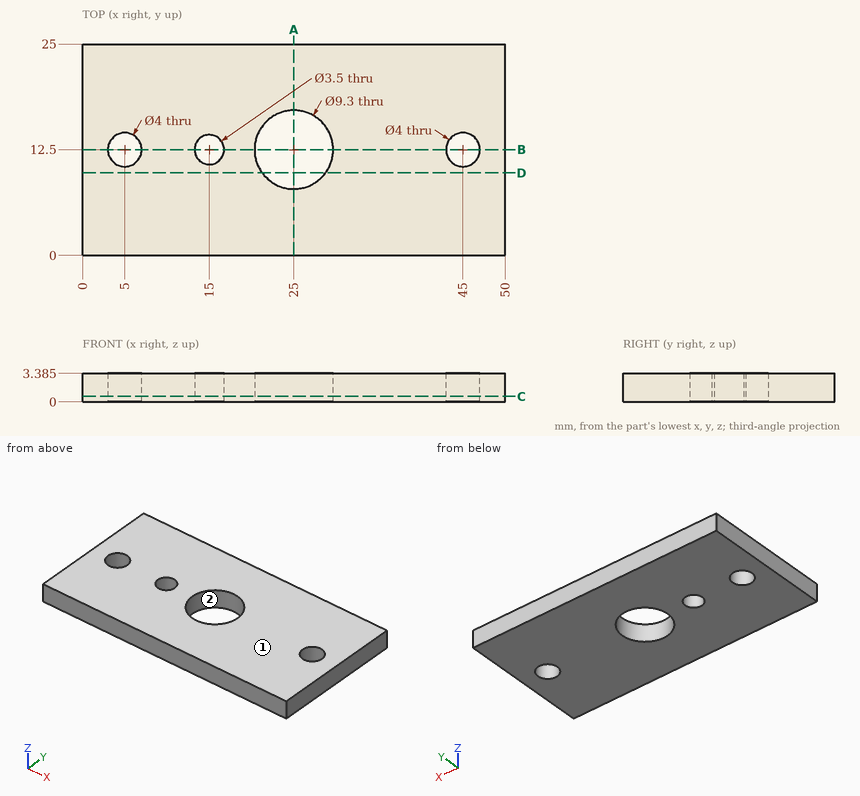
Check sheet for the drawn part. Datum: minimum x, y, z corner. Units: mm. Coordinates: 2 decimals unless noted, no trailing zeros. Order: outer loops, then holes, each group sorted by start corner. A loop starts at its lowest first (then second) coordinate and runs counter-clockwise, first axis right, second up. Notation, with made-up numbers: M 83.5,-7.75 L 132.5,-7.75 A13 cw 132.5,-3.75 Z; hole C -37,-40 d11. An arc over 180 degrees is marked long. One line per item, written item: value. Start each with the question number.
Item 1: Mould release check, pull along X, two halves, no side actions. Record for the marked faces 1 and 2: released by +X, released by -X, zero draft, split by the parting line, or undercut.
Item 2: Sectioned sample at C-C (z = 0.65). Enter the section's corners in (x, y), then the cut area to 3 significant figures.
Item 3: Gauge pin test, flat end, axial feed: pin 1 (5.5 mm diameter, centred on x = 15, y = 12.5, fed in from -Z). Record the tip position at first contact, or that the pin passes through.
Item 4: Sectioned sample at B-B (y = 12.5). Enter the section's corners in (x, z) (3 decimals), then the cut area to 3 significant figures.
Item 5: Sectioned sample at A-A (x = 25). Enter the section's corners in (y, z) (3 decimals), then the cut area to 3 significant figures.
Item 6: Sectioned sample at D-D (y = 9.75). Enter the section's corners in (x, z) (3 decimals).
Item 7: Scan lines: probe 1 along Y at (x, z) = (45, 1.6); probe 2 along Y at (x, z) = (15, 1.3); probe 3 along X at (y, z) = (13.5, 3.1). Record each from-to range of solid material in increasing order.
Conclusion:
1. face 1: zero draft
1. face 2: undercut
2. outline: M 0,0 L 50,0 L 50,25 L 0,25 Z; hole C 5,12.5 d4; hole C 15,12.5 d3.5; hole C 25,12.5 d9.3; hole C 45,12.5 d4
2. area: 1,150 mm^2
3. pin 1: stops at z = 0
4. outline: M 0,0 L 3,0 L 3,3.385 L 0,3.385 Z; M 7,0 L 13.25,0 L 13.25,3.385 L 7,3.385 Z; M 16.75,0 L 20.35,0 L 20.35,3.385 L 16.75,3.385 Z; M 29.65,0 L 43,0 L 43,3.385 L 29.65,3.385 Z; M 47,0 L 50,0 L 50,3.385 L 47,3.385 Z
4. area: 98.8 mm^2
5. outline: M 0,0 L 7.85,0 L 7.85,3.385 L 0,3.385 Z; M 17.15,0 L 25,0 L 25,3.385 L 17.15,3.385 Z
5. area: 53.1 mm^2
6. outline: M 0,0 L 21.25,0 L 21.25,3.385 L 0,3.385 Z; M 28.75,0 L 50,0 L 50,3.385 L 28.75,3.385 Z
7. probe 1: y = 0 to 10.5, 14.5 to 25
7. probe 2: y = 0 to 10.75, 14.25 to 25
7. probe 3: x = 0 to 3.27, 6.73 to 13.56, 16.44 to 20.46, 29.54 to 43.27, 46.73 to 50
